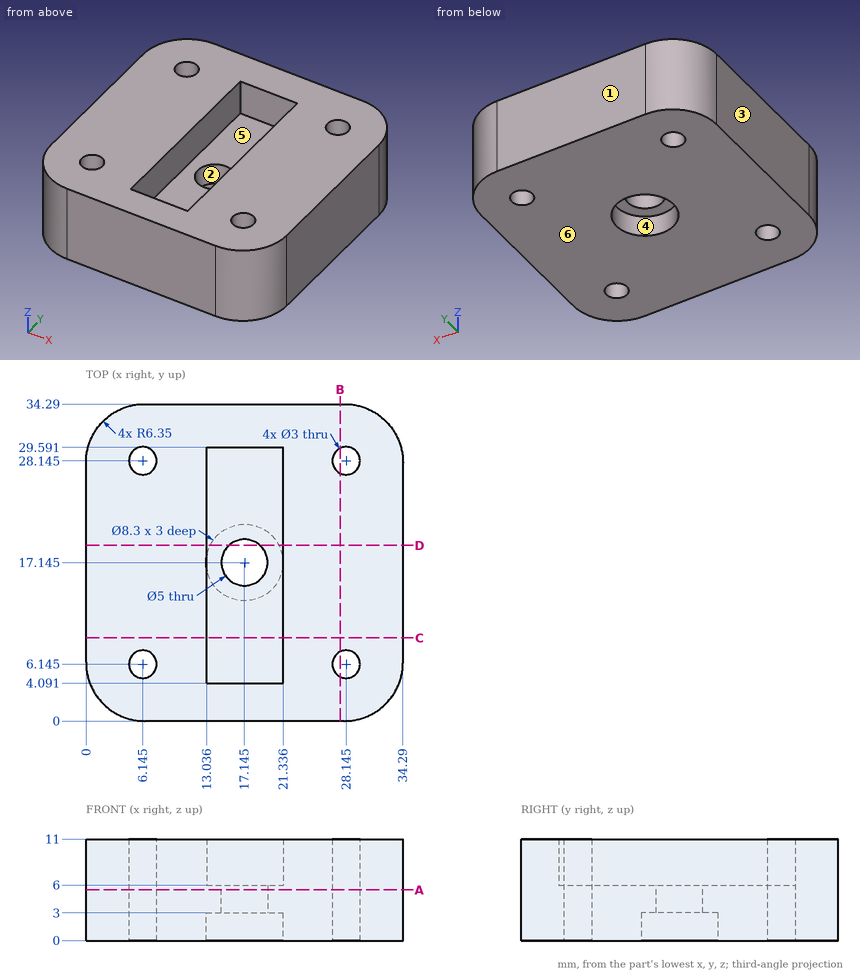
Input: dimensioned drawing with shaded views. Units: mm. Origin: part minimum x, y, z. A direction names the side the tool comes from. Give positions to 0.01 mm unless a question says otherwise; leave off trailing zeros. Order: outer loops, then holes, each group sorted by start corner. A loop starts at its lowest first (then second) coordinate and runs counter-clockwise, first axis right, second up. Notation, with made-up numbers: (69.5, 51.5) -> (81.5, 51.5) arc R19 ccw to (81.5, 77.5) -> close; hole circle Ø1 at (37, 27). An arc over 180 degrees is marked (long way). Use a Markdown table: item, result.
1) Ray query, line 1 along Y through (x, z) = (15, 9.5); line 2 along X through (y, z) = (13.5, 7); line 3 along Y through (x, z) = (28.5, 6.75). Return the intervals inside material, ascending. Write a range as [from, to].
Answer list:
| item | result |
|---|---|
| line 1 | [0, 4.09], [29.59, 34.29] |
| line 2 | [0, 13.04], [21.34, 34.29] |
| line 3 | [0.02, 4.69], [7.6, 26.69], [29.6, 34.27] |
2) Section query D-D, the plane y = 19. Return the cut outline in (x, z).
Answer list:
| item | result |
|---|---|
| outline | (0, 0) -> (13.43, 0) -> (13.43, 3) -> (15.47, 3) -> (15.47, 6) -> (13.04, 6) -> (13.04, 11) -> (0, 11) -> close; (18.82, 3) -> (20.86, 3) -> (20.86, 0) -> (34.29, 0) -> (34.29, 11) -> (21.34, 11) -> (21.34, 6) -> (18.82, 6) -> close |
3) Section query C-C, the plane y = 9. Return the cut outline in (x, z), then the cut area to 3 significant figures.
Answer list:
| item | result |
|---|---|
| outline | (0, 0) -> (34.29, 0) -> (34.29, 11) -> (21.34, 11) -> (21.34, 6) -> (13.04, 6) -> (13.04, 11) -> (0, 11) -> close |
| area | 336 mm² |
4) Contact query for a flat-ended pin moving along its axis: P1, Ø4, axis at x = 18.5, y = 18, coming from the -Z side. Output: stop coordinate, or through.
Answer list:
| item | result |
|---|---|
| P1 | z = 3 |
5) Section query A-A, the plane z = 5.5. Return the cut outline in (x, y) (3 decimals).
Answer list:
| item | result |
|---|---|
| outline | (0, 6.35) arc R6.35 ccw to (6.35, 0) -> (27.94, 0) arc R6.35 ccw to (34.29, 6.35) -> (34.29, 27.94) arc R6.35 ccw to (27.94, 34.29) -> (6.35, 34.29) arc R6.35 ccw to (0, 27.94) -> close; hole circle Ø3 at (6.145, 6.145); hole circle Ø3 at (6.145, 28.145); hole circle Ø5 at (17.145, 17.145); hole circle Ø3 at (28.145, 6.145); hole circle Ø3 at (28.145, 28.145) |
6) Reachability of the marked faces 4, 5 and 6 from +Z, -Z, +X, -X, +Y, -Y: full face, straight path, thin tool, end or side. Return the list, or none.
Answer list:
| item | result |
|---|---|
| face 4 | -Z |
| face 5 | +Z |
| face 6 | -Z, +X, -X, +Y, -Y |
7) Mould query, pull axis Y, two halves, no side actions, for the marked faces 1, 2 and 3. Classes: +Y half, -Y half, draft (parallel to the pull), parting line (faces both ways), or undercut.
Answer list:
| item | result |
|---|---|
| face 1 | +Y half |
| face 2 | undercut |
| face 3 | draft |
8) Section query B-B, the plane x = 27.5. Return the cut outline in (y, z), then the cut area to 3 significant figures.
Answer list:
| item | result |
|---|---|
| outline | (0, 0) -> (4.79, 0) -> (4.79, 11) -> (0, 11) -> close; (7.5, 0) -> (26.79, 0) -> (26.79, 11) -> (7.5, 11) -> close; (29.5, 0) -> (34.29, 0) -> (34.29, 11) -> (29.5, 11) -> close |
| area | 318 mm² |
